Check sheet for the modelled part. Datum: model origin and axes. Units: mm. A direction names the side the tool comes from. Round coordinates to 2 decimals unless told otherwise and drop trailing zeros. Write each loop counter-clockwise with the first axis right and the second up, starting at its lowest first coordinate (ties: lowest second). Pieces come first, ordered by that corner, then holes. Notation, with made-up numbers: (79, 65.25) -> (137, 65.25) arc R22 ccw to (137, 99.25) -> close; hole circle Ø8 at (66.25, -38). An arc over 180 degrees is marked (long way). One line per item, written item: value. Start each with the question number.
Autodesk Inventor part; units mm, degrees
ref_plane "작업 평면3" through (0, 2.2, 0) normal (0, -1, 0) x (1, 0, 0)
ref_plane "YZ Plane" through (0, 0, 0) normal (1, 0, 0) x (0, 1, 0)
ref_plane "XZ Plane" through (0, 0, 0) normal (0, 1, 0) x (-1, 0, 0)
sketch "스케치1" plane through (0, 0, 0) normal (0, 1, 0) x (-1, 0, 0)
  line L0 (-16.2959, 6.75) -> (-6.75, 16.2959)
  line L1 (-6.75, 16.2959) -> (6.75, 16.2959)
  line L2 (6.75, 16.2959) -> (16.2959, 6.75)
  line L3 (16.2959, 6.75) -> (16.2959, -6.75)
  line L4 (16.2959, -6.75) -> (6.75, -16.2959)
  line L5 (6.75, -16.2959) -> (-6.75, -16.2959)
  line L6 (-6.75, -16.2959) -> (-16.2959, -6.75)
  line L7 (-16.2959, -6.75) -> (-16.2959, 6.75)
  line L8 (19.4959, 8.0755) -> (19.4959, -8.0755)
  line L9 (19.4959, -8.0755) -> (8.0755, -19.4959)
  line L10 (8.0755, -19.4959) -> (-8.0755, -19.4959)
  line L11 (-8.0755, -19.4959) -> (-19.4959, -8.0755)
  line L12 (-19.4959, -8.0755) -> (-19.4959, 8.0755)
  line L13 (-19.4959, 8.0755) -> (-8.0755, 19.4959)
  line L14 (-8.0755, 19.4959) -> (8.0755, 19.4959)
  line L15 (8.0755, 19.4959) -> (19.4959, 8.0755)
  point P0 (0, 0)
  point P1 (0, 0)
  point P2 (0, 0)
  dimension "d0" = 13.5
  dimension "d1" = 3.2
extrude "돌출1" add sketch "스케치1" along normal blind 4.4 contours L0 L1 L2 L3 L4 L5 L6 L7 | L8 L9 L10 L11 L12 L13 L14 L15
sketch "스케치14" plane through (0, 4.4, 0) normal (0, 1, 0) x (1, 0, 0)
  line L0 (6.5843, -15.8959) -> (-6.5843, -15.8959)
  line L1 (-6.5843, -15.8959) -> (-15.8959, -6.5843)
  line L2 (-15.8959, -6.5843) -> (-15.8959, 6.5843)
  line L3 (-15.8959, 6.5843) -> (-6.5843, 15.8959)
  line L4 (-6.5843, 15.8959) -> (6.5843, 15.8959)
  line L5 (6.5843, 15.8959) -> (15.8959, 6.5843)
  line L6 (15.8959, 6.5843) -> (15.8959, -6.5843)
  line L7 (15.8959, -6.5843) -> (6.5843, -15.8959)
  line L8 (-7.4127, 17.8959) -> (7.4127, 17.8959)
  line L9 (7.4127, 17.8959) -> (17.8959, 7.4127)
  line L10 (17.8959, 7.4127) -> (17.8959, -7.4127)
  line L11 (17.8959, -7.4127) -> (7.4127, -17.8959)
  line L12 (7.4127, -17.8959) -> (-7.4127, -17.8959)
  line L13 (-7.4127, -17.8959) -> (-17.8959, -7.4127)
  line L14 (-17.8959, -7.4127) -> (-17.8959, 7.4127)
  line L15 (-17.8959, 7.4127) -> (-7.4127, 17.8959)
  line L16 (19.4959, -8.0755) -> (19.4959, 8.0755)
  point P0 (0, 0)
  point P1 (0, 0)
  point P2 (0, 0)
  dimension "d138" = 2
  dimension "d139" = 1.6
extrude "돌출16" cut sketch "스케치14" against normal blind 1.2
sketch "스케치15" plane through (0, 4.4, 0) normal (0, 1, 0) x (1, 0, 0)
  line L0 (-15.8959, -6.5843) -> (-6.5843, -15.8959)
  line L1 (-6.5843, -15.8959) -> (6.5843, -15.8959)
  line L2 (6.5843, -15.8959) -> (15.8959, -6.5843)
  line L3 (15.8959, -6.5843) -> (15.8959, 6.5843)
  line L4 (15.8959, 6.5843) -> (6.5843, 15.8959)
  line L5 (6.5843, 15.8959) -> (-6.5843, 15.8959)
  line L6 (-6.5843, 15.8959) -> (-15.8959, 6.5843)
  line L7 (-15.8959, 6.5843) -> (-15.8959, -6.5843)
  point P0 (0, 0)
extrude "돌출17" cut sketch "스케치15" against normal blind 0.6
sketch "스케치16" plane through (0, 3.8, 0) normal (0, 1, 0) x (1, 0, 0)
  line L0 (-5.9216, 14.2959) -> (5.9216, 14.2959)
  line L1 (5.9216, 14.2959) -> (14.2959, 5.9216)
  line L2 (14.2959, 5.9216) -> (14.2959, -5.9216)
  line L3 (14.2959, -5.9216) -> (5.9216, -14.2959)
  line L4 (5.9216, -14.2959) -> (-5.9216, -14.2959)
  line L5 (-5.9216, -14.2959) -> (-14.2959, -5.9216)
  line L6 (-14.2959, -5.9216) -> (-14.2959, 5.9216)
  line L7 (-14.2959, 5.9216) -> (-5.9216, 14.2959)
  line L8 (15.8959, 6.5843) -> (15.8959, -6.5843)
  point P0 (0, 0)
  point P1 (0, 0)
  dimension "d144" = 1.6
extrude "돌출18" cut sketch "스케치16" against normal up to surface (3.8 mm away)
fillet "모깎기2" radius 1.2 16 edges at (0, 4.4, -19.4959) (-13.7857, 4.4, -13.7857) (13.7857, 4.4, -13.7857) (19.4959, 4.4, 0) (13.7857, 4.4, 13.7857) (0, 4.4, 19.4959) (-13.7857, 4.4, 13.7857) (-19.4959, 4.4, 0) (-19.4959, 0, 0) (-13.7857, 0, 13.7857) (0, 0, 19.4959) (13.7857, 0, 13.7857) (-13.7857, 0, -13.7857) (0, 0, -19.4959) (19.4959, 0, 0) (13.7857, 0, -13.7857)
ref_plane "작업 평면3" through (0, 2.2, 0) normal (0, -1, 0) x (1, 0, 0)
mirror "미러6" about plane through (0, 2.2, 0) normal (0, -1, 0) of "돌출17", "돌출16"
properties part number "OV-PAM_ring_2"
1. Access from +Z, -Z, +X, -X, +Y, -Y to the whole of each face (thin tool, end or side, straight path). Record for faces 1 (the face through (11.17, 0.9, 11.31)), 2 (the face through (11, 3.8, 11)), 3 (the face through (0, 2, -14.296)), 4 (the face through (-19.135, 0.342, -0.113)).
2. Cross-section at C-C (y = 2.6). Record the cut outline in (x, z).
3. Material ranges on probe 1 along X at (y, z) = (0.9, -12); probe 2 along Z at (x, y) = (-1.5, 1.9); probe 3 along Z at (x, y) = (-3, 0.9), recorded low to high.
4. Depth check by flat-ended pin: pin 1 Ø4 at (x, z) = (-15.5, 3) entering from +Y; pin 2 Ø0.6 at (y, z) = (0.5, -2.5) entering from +X; pin 3 Ø1.5 at (y, z) = (1.5, -11.5) entering from -X; pin 4 Ø0.7 at (x, y) = (-1, 3.5) entering from +Z. Enter the tip coordinate at first touch or a pass-through.
5. Cross-section at B-B (z = -5). Record the cut outline in (x, y).
6. Cross-section at A-A (x = -2). Record the cut outline in (y, z).
7. Release check for a two-part mould opening along Z. For faces 5 (the face through (-13.706, 2.186, 13.866)), 6 (the face through (-12.1, 4.4, -13.5)), 7 (the face through (-10.05, 2.22, 10.17)) record: +Z half, -Z half, draft (parallel to the pull), parting line (faces both ways), or undercut.
Working result:
1. face 1: -Y
1. face 2: +Y
1. face 3: +Y, -Y
1. face 4: +Z, -Z, -X, -Y
2. outline: (-19.5, -8.08) -> (-8.08, -19.5) -> (8.08, -19.5) -> (19.5, -8.08) -> (19.5, 8.08) -> (8.08, 19.5) -> (-8.08, 19.5) -> (-19.5, 8.08) -> close; hole (-14.3, -5.92) -> (-5.92, -14.3) -> (5.92, -14.3) -> (14.3, -5.92) -> (14.3, 5.92) -> (5.92, 14.3) -> (-5.92, 14.3) -> (-14.3, 5.92) -> close
3. probe 1: x = -15.52 to -13.31, -10.48 to -8.22, 8.22 to 10.48, 13.31 to 15.52
3. probe 2: z = -19.5 to -14.3, 14.3 to 19.5
3. probe 3: z = -19.46 to -17.9, -15.9 to -14.3, 14.3 to 15.9, 17.9 to 19.46
4. pin 1: stops at y = 3.8
4. pin 2: stops at x = 19.43
4. pin 3: stops at x = -16.82
4. pin 4: stops at z = 19.5
5. outline: (-19.5, 1.2) arc R1.2 ccw to (-18.3, 0) -> (-17.9, 0) -> (-17.9, 1.2) -> (-15.9, 1.2) -> (-15.9, 0.6) -> (-14.3, 0.6) -> (-14.3, 3.8) -> (-15.9, 3.8) -> (-15.9, 3.2) -> (-17.9, 3.2) -> (-17.9, 4.4) -> (-18.3, 4.4) arc R1.2 ccw to (-19.5, 3.2) -> close; (14.3, 0.6) -> (15.9, 0.6) -> (15.9, 1.2) -> (17.9, 1.2) -> (17.9, 0) -> (18.3, 0) arc R1.2 ccw to (19.5, 1.2) -> (19.5, 3.2) arc R1.2 ccw to (18.3, 4.4) -> (17.9, 4.4) -> (17.9, 3.2) -> (15.9, 3.2) -> (15.9, 3.8) -> (14.3, 3.8) -> close
6. outline: (0, -18.3) arc R1.2 ccw to (1.2, -19.5) -> (3.2, -19.5) arc R1.2 ccw to (4.4, -18.3) -> (4.4, -17.9) -> (3.2, -17.9) -> (3.2, -15.9) -> (3.8, -15.9) -> (3.8, -14.3) -> (0.6, -14.3) -> (0.6, -15.9) -> (1.2, -15.9) -> (1.2, -17.9) -> (0, -17.9) -> close; (0, 17.9) -> (1.2, 17.9) -> (1.2, 15.9) -> (0.6, 15.9) -> (0.6, 14.3) -> (3.8, 14.3) -> (3.8, 15.9) -> (3.2, 15.9) -> (3.2, 17.9) -> (4.4, 17.9) -> (4.4, 18.3) arc R1.2 ccw to (3.2, 19.5) -> (1.2, 19.5) arc R1.2 ccw to (0, 18.3) -> close
7. face 5: +Z half
7. face 6: draft
7. face 7: undercut
